Read the model definition and answer for the solid it produces. Units are mm, in the model's axes. A direction names the side the tool comes from. Round coordinates to 2 decimals unless told otherwise and drop trailing zeros. Write each loop counter-clockwise with the first axis right and the second up, starting at its lowest first coordinate (ties: lowest second). Pieces come first, ordered by that corner, then holes. Notation, with made-up numbers: (54, 57.5) -> (72, 57.5) arc R23 ccw to (72, 87.5) -> close; hole circle Ø10 at (19, 39.25). An arc over 180 degrees is marked (long way). Return JSON: item names as keys, results as strings.
from build123d import *

# Parameters (mm, degrees)
SKETCH3_R           = 3.4
BOSS_EXTRUDE1_DEPTH = 100
CUT_EXTRUDE1_DEPTH  = 38
CUT_EXTRUDE2_DEPTH  = 38


with BuildPart() as part:
    # Sketch3 → Boss-Extrude1 (new body)
    with BuildSketch(Plane.XY):
        Polygon((-4.1, 2.544365081), (-4.1, -2.544365081), (-10.463961031, -8.908326112), (-13.02814489, -8.908326112), (-13.02814489, -5.726345597), (-15, -5.726345597), (-15, -15), (-5.726345597, -15), (-5.726345597, -13.02814489), (-8.908326112, -13.02814489), (-8.908326112, -10.463961031), (-2.544365081, -4.1), (2.544365081, -4.1), (8.908326112, -10.463961031), (8.908326112, -13.02814489), (5.726345597, -13.02814489), (5.726345597, -15), (15, -15), (15, -5.726345597), (13.02814489, -5.726345597), (13.02814489, -8.908326112), (10.463961031, -8.908326112), (4.1, -2.544365081), (4.1, 2.544365081), (10.463961031, 8.908326112), (13.02814489, 8.908326112), (13.02814489, 5.726345597), (15, 5.726345597), (15, 15), (5.726345597, 15), (5.726345597, 13.02814489), (8.908326112, 13.02814489), (8.908326112, 10.463961031), (2.544365081, 4.1), (-2.544365081, 4.1), (-8.908326112, 10.463961031), (-8.908326112, 13.02814489), (-5.726345597, 13.02814489), (-5.726345597, 15), (-15, 15), (-15, 5.726345597), (-13.02814489, 5.726345597), (-13.02814489, 8.908326112), (-10.463961031, 8.908326112), align=None)
        Circle(SKETCH3_R, mode=Mode.SUBTRACT)
    extrude(amount=BOSS_EXTRUDE1_DEPTH)

    # Sketch4 → Cut-Extrude1 (cut)
    with BuildSketch(Plane(origin=(0, 15, 0), x_dir=(1, 0, 0), z_dir=(0, 1, 0))):
        Polygon((-15, -100), (15, -100), (15, -87.573593129), align=None)
    extrude(amount=-CUT_EXTRUDE1_DEPTH, mode=Mode.SUBTRACT)

    # Sketch5 → Cut-Extrude2 (cut)
    with BuildSketch(Plane(origin=(0, 15, 0), x_dir=(1, 0, 0), z_dir=(0, 1, 0))):
        Polygon((-15, 0), (15, 0), (15, -12.426406871), align=None)
    extrude(amount=-CUT_EXTRUDE2_DEPTH, mode=Mode.SUBTRACT)


solid = part.part
Item 1: Section C-C (x = 0) is taken. Give the vertices of the cut face in (y, z).
Worked answers:
{"outline": "(-4.1, 6.21) -> (-3.4, 6.21) -> (-3.4, 93.79) -> (-4.1, 93.79) -> close; (3.4, 6.21) -> (4.1, 6.21) -> (4.1, 93.79) -> (3.4, 93.79) -> close"}
Item 2: For a pull along Y with two mould halves and no side action, classify faces 1 (the flat face through (-12, 8.908, 49)), 2 (the flat face through (-10, -15, 49)), 3 (the flat face through (7, 13.028, 49)), 4 (the flat face through (3.54, 3.54, 7.68)) as released by +Y, released by -Y, zero draft, split by the parting line, or undercut.
Worked answers:
{"face 1": "undercut", "face 2": "released by -Y", "face 3": "undercut", "face 4": "zero draft"}
Item 3: Section A-A (x = -7) is taken. Give the vertices of the cut face in (y, z).
Worked answers:
{"outline": "(-15, 3.31) -> (-13.03, 3.31) -> (-13.03, 96.69) -> (-15, 96.69) -> close; (-8.56, 3.31) -> (-5.44, 3.31) -> (-5.44, 96.69) -> (-8.56, 96.69) -> close; (5.44, 3.31) -> (8.56, 3.31) -> (8.56, 96.69) -> (5.44, 96.69) -> close; (13.03, 3.31) -> (15, 3.31) -> (15, 96.69) -> (13.03, 96.69) -> close"}
Item 4: A tool of negligible diameter and unlimited length cuts with its end or side. For faces 5 (the flat face through (0, 4.1, 49)), 6 (the flat face through (5.726, -14, 49)), 7 (the flat face through (-8.908, 12, 49)), 8 (the flat face through (14, -5.726, 49)), from which of +Z, -Z, +X, -X, +Y, -Y can it reach the whole face along a straight path? Write none if from no direction.
Worked answers:
{"face 5": "+Z, -Z, +Y", "face 6": "+Z, -Z, -Y", "face 7": "+Z, -Z", "face 8": "+Z, -Z, +X"}
Item 5: Flat-ended cylindrical pins translate along their axes: pin 1 (1.5 mm diameter, centred on y = -3, z = 22, fed in from -X); pin 2 (1 mm diameter, centred on x = -7, y = -9, fed in from +Z); pin 3 (10 mm diameter, centred on x = 0, z = 55, fed in from -Y). Find the tip coordinate at first contact, or state that the pin passes through.
Worked answers:
{"pin 1": "stops at x = -5.31", "pin 2": "stops at z = 96.89", "pin 3": "stops at y = -6.56"}
Item 6: Section B-B (y = 0) is taken. Give the vertices of the cut face in (x, z), then the cut area to 3 significant figures.
Worked answers:
{"outline": "(-4.1, 4.51) -> (-3.4, 4.8) -> (-3.4, 95.2) -> (-4.1, 95.49) -> close; (3.4, 7.62) -> (4.1, 7.91) -> (4.1, 92.09) -> (3.4, 92.38) -> close", "area": "123 mm2"}
Item 7: Straight lines are drawn through the part: L1, parallel to Y at x = 0, z = 40; L2, parallel to X at y = -7.5, z = 35. For each, find the intervals that lie inside material, in ascending order. Write a range as [from, to].
Worked answers:
{"L1": "y = [-4.1, -3.4], [3.4, 4.1]", "L2": "x = [-15, -13.03], [-9.06, -5.94], [5.94, 9.06], [13.03, 15]"}
